```python
from build123d import *

# Parameters (mm, degrees)
SKETCH1_W             = 100
SKETCH1_H             = 10
BOSS_EXTRUDE1_DEPTH   = 50
BOSS_EXTRUDE2_DEPTH   = 25
BOSS_EXTRUDE2_2_DEPTH = 25
SKETCH1_7_W           = 5
SKETCH1_7_H           = 14.963037634
BOSS_EXTRUDE3_DEPTH   = 12.5
BOSS_EXTRUDE4_DEPTH   = 6.25
BOSS_EXTRUDE5_DEPTH   = 12.5


with BuildPart() as part:
    # Sketch1 → Boss-Extrude1 (new body)
    with BuildSketch(Plane.XY):
        with Locations((6.905913978, -26.92641129)):
            Rectangle(SKETCH1_W, SKETCH1_H)
    extrude(amount=BOSS_EXTRUDE1_DEPTH)



with BuildPart() as body_2:
    # Sketch1_6 → Boss-Extrude2 (new body)
    with BuildSketch(Plane.XY):
        Polygon((-18.131048387, 3.036626344), (-18.131048387, -6.963373656), (-13.131048387, -6.963373656), (-8.131048387, -6.963373656), (-8.131048387, 3.036626344), align=None)
    extrude(amount=BOSS_EXTRUDE2_DEPTH)


with BuildPart() as body_3:
    # Sketch1_6 → Boss-Extrude2 2 (new body)
    with BuildSketch(Plane.XY):
        Polygon((26.868951613, -6.963373656), (31.868951613, -6.963373656), (31.868951613, 3.036626344), (21.868951613, 3.036626344), (21.868951613, -6.963373656), align=None)
    extrude(amount=BOSS_EXTRUDE2_2_DEPTH)


with BuildPart() as part_1:
    add(part.part)

    add(body_2.part)  # Boss-Extrude3 merges body 2

    add(body_3.part)  # Boss-Extrude3 merges body 3
    # Sketch1_7 → Boss-Extrude3 (add)
    with BuildSketch(Plane.XY):
        with Locations((-15.631048387, -14.444892473)):
            Rectangle(SKETCH1_7_W, SKETCH1_7_H)
        with Locations((29.368951613, -14.444892473)):
            Rectangle(SKETCH1_7_W, SKETCH1_7_H)
    extrude(amount=BOSS_EXTRUDE3_DEPTH)

    # Sketch1_8 → Boss-Extrude4 (add)
    with BuildSketch(Plane.XY):
        with BuildLine():
            Line((-13.131048387, -6.963373656), (-13.131048387, -21.92641129))
            Line((-13.131048387, -21.92641129), (26.868951613, -21.92641129))
            Line((26.868951613, -21.92641129), (26.868951613, -6.963373656))
            Line((26.868951613, -6.963373656), (21.868951613, -6.963373656))
            Line((21.868951613, -6.963373656), (21.868951613, 3.036626344))
            Line((21.868951613, 3.036626344), (16.868951613, 3.036626344))
            Line((16.868951613, 3.036626344), (11.868951613, 3.036626344))
            ThreePointArc((11.868951613, 3.036626344), (6.868951613, -1.963373656), (1.868951613, 3.036626344))
            Line((1.868951613, 3.036626344), (-3.131048387, 3.036626344))
            Line((-3.131048387, 3.036626344), (-8.131048387, 3.036626344))
            Line((-8.131048387, 3.036626344), (-8.131048387, -6.963373656))
            Line((-8.131048387, -6.963373656), (-13.131048387, -6.963373656))
        make_face()
        with BuildLine():
            ThreePointArc((31.868951613, 3.036626344), (6.868951613, 28.036626344), (-18.131048387, 3.036626344))
            Line((-18.131048387, 3.036626344), (-8.131048387, 3.036626344))
            Line((-8.131048387, 3.036626344), (-3.131048387, 3.036626344))
            ThreePointArc((-3.131048387, 3.036626344), (6.868951613, 13.036626344), (16.868951613, 3.036626344))
            Line((16.868951613, 3.036626344), (21.868951613, 3.036626344))
            Line((21.868951613, 3.036626344), (31.868951613, 3.036626344))
        make_face()
    extrude(amount=BOSS_EXTRUDE4_DEPTH)

    # Sketch1_9 → Boss-Extrude5 (add)
    with BuildSketch(Plane.XY):
        with BuildLine():
            ThreePointArc((31.868951613, 3.036626344), (6.868951613, 28.036626344), (-18.131048387, 3.036626344))
            Line((-18.131048387, 3.036626344), (-8.131048387, 3.036626344))
            Line((-8.131048387, 3.036626344), (-3.131048387, 3.036626344))
            ThreePointArc((-3.131048387, 3.036626344), (6.868951613, 13.036626344), (16.868951613, 3.036626344))
            Line((16.868951613, 3.036626344), (21.868951613, 3.036626344))
            Line((21.868951613, 3.036626344), (31.868951613, 3.036626344))
        make_face()
    extrude(amount=-BOSS_EXTRUDE5_DEPTH)


solid = part_1.part
```
Part model, mm, in its own coordinate system. A direction names the side the tool comes from. Round coordinates to 2 decimals unless told otherwise and drop trailing zeros. Loops run counter-clockwise (first coordinate to the right, second up) from the corner with the lowest first, then second, coordinate; pieces in that order, holes last. Notation, with made-up numbers: (-38, 10.5) -> (-17, 10.5) arc R32 ccw to (-17, 45.5) -> close; hole circle Ø3 at (13.5, -3). An arc over 180 degrees is marked (long way). Use one line per item in the form item = value. Start each with the question number.
Item 1: Band-saw the part on B-B (y = 5.5). List the corners of the cut face in (x, z), plus the area to 3 significant figures.
Item 2: Band-saw the part on D-D (z = 10). List the corners of the cut face in (x, y).
Item 3: Band-saw the part on C-C (x = -6). List the corners of the cut face in (y, z), plus the area to 3 significant figures.
Item 4: Band-saw the part on A-A (z = 16.5). List the corners of the cut face in (x, y).
Item 5: Drop flat-ended pins along their axis: pin 1 Ø11 at (y, z) = (-2.5, 20.5) entering from -X; pin 2 Ø1.9 at (y, z) = (-16, 10.5) entering from +X; pin 3 Ø8 at (x, y) = (29, -2.5) entering from +Z. Give the stop position or say it passes through.
Item 6: Tool access for faces 1 (the flat face through (-8.131, -2, 15)), 2 (the flat face through (-11, 3.037, -6)), 3 (the flat face through (14, 3.037, 3)): list every direction of +Z, -Z, +X, -X, +Y, -Y with a clear straight run to the whole face (end or side of a thin tool).
Item 7: Drill centre lines: line 1 along Y through (x, z) = (38.5, 43); line 2 along X through (y, z) = (-13.5, 8); line 3 along Z through (x, y) = (-10, 11). Where is each one in solid material? Low to high.
Item 8: Two-plate mould, pull along X, no slides. Class faces 4 (the flat face through (-13, 3.037, 15)), 5 (the flat face through (31.869, -7, 10)), 6 (the cylindrical face through (6.979, -1.962, 3.081)): released by +X, released by -X, zero draft, split by the parting line, or undercut.
Data:
q1.outline = (-18.01, -12.5) -> (-2.82, -12.5) -> (-2.82, 6.25) -> (-18.01, 6.25) -> close; (16.56, -12.5) -> (31.75, -12.5) -> (31.75, 6.25) -> (16.56, 6.25) -> close
q1.area = 569 mm^2
q2.outline = (-43.09, -31.93) -> (56.91, -31.93) -> (56.91, -21.93) -> (31.87, -21.93) -> (31.87, 3.04) -> (21.87, 3.04) -> (21.87, -6.96) -> (26.87, -6.96) -> (26.87, -21.93) -> (-13.13, -21.93) -> (-13.13, -6.96) -> (-8.13, -6.96) -> (-8.13, 3.04) -> (-18.13, 3.04) -> (-18.13, -21.93) -> (-43.09, -21.93) -> close
q3.outline = (-31.93, 0) -> (3.04, 0) -> (3.04, -12.5) -> (24.47, -12.5) -> (24.47, 6.25) -> (-21.93, 6.25) -> (-21.93, 50) -> (-31.93, 50) -> close
q3.area = 1,060 mm^2
q4.outline = (-43.09, -31.93) -> (56.91, -31.93) -> (56.91, -21.93) -> (-43.09, -21.93) -> close; (-18.13, -6.96) -> (-8.13, -6.96) -> (-8.13, 3.04) -> (-18.13, 3.04) -> close; (21.87, -6.96) -> (31.87, -6.96) -> (31.87, 3.04) -> (21.87, 3.04) -> close
q5.pin_1 = -18.13
q5.pin_2 = 31.87
q5.pin_3 = 25
q6.face_1 = +Z, +Y
q6.face_2 = -Z, +X, -X, -Y
q6.face_3 = +Z, -Z
q7.line_1 = -31.93 to -21.93
q7.line_2 = -18.13 to -13.13, 26.87 to 31.87
q7.line_3 = -12.5 to 6.25
q8.face_4 = zero draft
q8.face_5 = released by +X
q8.face_6 = undercut
